For this review, take the finished solid that the model builds, in its own axes (mm). A direction names the side the tool comes from. Round coordinates to 2 decimals unless told otherwise and drop trailing zeros. Order: outer loops, then holes, each group sorted by start corner. A loop starts at its lowest first (then second) coordinate and runs counter-clockwise, first axis right, second up. Notation, with made-up numbers: (50.25, -5) - (63.25, -5) arc R20 ccw to (63.25, 13) - close; hole circle Ø5 at (66.25, 17). An arc over 180 degrees is marked (long way). Write each question's results on one line, items separated by ' | '. Start each with the question number.
(1) Insertion check: pin 1 Ø6.5 at (x, y) = (-8, 31) entering from +Z. The pin has a flat end and moves straight along its axis. Give the tip position at first contact, or say it passes through.
(2) Draft analysis for pull direction Y (two halves, no side actions). For faces 4 (the flat face through (69.574, 7, 22)), 5 (the flat face through (-1, -33.728, 29)), 6 (the cylindrical face through (65.846, 7.784, 31.661)), state which applies: pulls with the +Y half, pulls with the -Y half, needs draft (parallel to the pull), parting line crosses it, or undercut.
(3) Take a section at A-A, the plane x = -31. Give the boundary of the cut face in (y, z).
(4) Take a section at B-B, the plane y = 0. Give the boundary of the cut face in (x, z), plus the area to 3 significant figures.
(5) For faces 1 (the flat face through (-1, 25.561, 30)), 2 (the flat face through (24.2, 30, 50)), 3 (the cylindrical face through (-65.74, 7.784, 31.661)), list the 3-axis set-ups (+Z, -Z, +X, -X, +Y, -Y) from which the entire face can be reached by the end or side of a thin tool; tool diameter is ignored.
(6) For L1, parallel to X at y = -30, z = 54.5; L2, parallel to Z at x = -64, y = 0; L3, parallel to X at y = 19.5, z = 33, list the stretches that pass through material, from the lowest coordinate up. Write a range as from..to.
(7) Take a section at D-D, the plane y = -16. Give the boundary of the cut face in (x, z).
(8) Take a section at C-C, the plane z = 29.21. Give the boundary of the cut face in (x, y).
```python
from build123d import *

# Parameters (mm, degrees)
F0_W     = 139.147832
F0_H     = 67.456446
F1_DEPTH = 58.42
F2_R     = 8.160902
F3_DEPTH = 139.148833
F4_W     = 124.023072
F4_H     = 51.121704
F5_DEPTH = 58.421
F6_W     = 51.424196
F6_H     = 16.221908
F7_DEPTH = 67.457447


with BuildPart() as f1:
    # F0 (on Top) → F1 (new body)
    with BuildSketch(Plane.XY):
        Rectangle(F0_W, F0_H)
    extrude(amount=F1_DEPTH)

    # F2 (on face) → F3 (cut, through all)
    with BuildSketch(Plane.YZ.offset(69.573916)):
        with Locations((0, 29.21)):
            Circle(F2_R)
    extrude(amount=-F3_DEPTH, mode=Mode.SUBTRACT)

    # F4 (on face) → F5 (cut, through all)
    with BuildSketch(Plane.XY.offset(58.42)):
        Rectangle(F4_W, F4_H)
    extrude(amount=-F5_DEPTH, mode=Mode.SUBTRACT)

    # F6 (on face) → F7 (cut, through all)
    with BuildSketch(Plane.XZ.offset(33.728223)):
        with Locations((-1.512476, 50.309046)):
            Rectangle(F6_W, F6_H)
    extrude(amount=-F7_DEPTH, mode=Mode.SUBTRACT)


solid = f1.part
```
Results below:
1) pin 1: stops at z = 42.2
2) face 4: needs draft | face 5: pulls with the -Y half | face 6: undercut
3) outline: (-33.73, 0) - (-25.56, 0) - (-25.56, 58.42) - (-33.73, 58.42) - close; (25.56, 0) - (33.73, 0) - (33.73, 58.42) - (25.56, 58.42) - close
4) outline: (-69.57, 0) - (-62.01, 0) - (-62.01, 21.05) - (-69.57, 21.05) - close; (-69.57, 37.37) - (-62.01, 37.37) - (-62.01, 58.42) - (-69.57, 58.42) - close; (62.01, 0) - (69.57, 0) - (69.57, 21.05) - (62.01, 21.05) - close; (62.01, 37.37) - (69.57, 37.37) - (69.57, 58.42) - (62.01, 58.42) - close | area: 637 mm^2
5) face 1: +Z, -Z | face 2: +Z, +Y, -Y | face 3: +X, -X
6) L1: x = -69.57..-27.22, 24.2..69.57 | L2: z = 0..21.05, 37.37..58.42 | L3: x = -69.57..-62.01, 62.01..69.57
7) outline: (-69.57, 0) - (-62.01, 0) - (-62.01, 58.42) - (-69.57, 58.42) - close; (62.01, 0) - (69.57, 0) - (69.57, 58.42) - (62.01, 58.42) - close
8) outline: (-69.57, -33.73) - (69.57, -33.73) - (69.57, -8.16) - (62.01, -8.16) - (62.01, -25.56) - (-62.01, -25.56) - (-62.01, -8.16) - (-69.57, -8.16) - close; (-69.57, 8.16) - (-62.01, 8.16) - (-62.01, 25.56) - (62.01, 25.56) - (62.01, 8.16) - (69.57, 8.16) - (69.57, 33.73) - (-69.57, 33.73) - close
